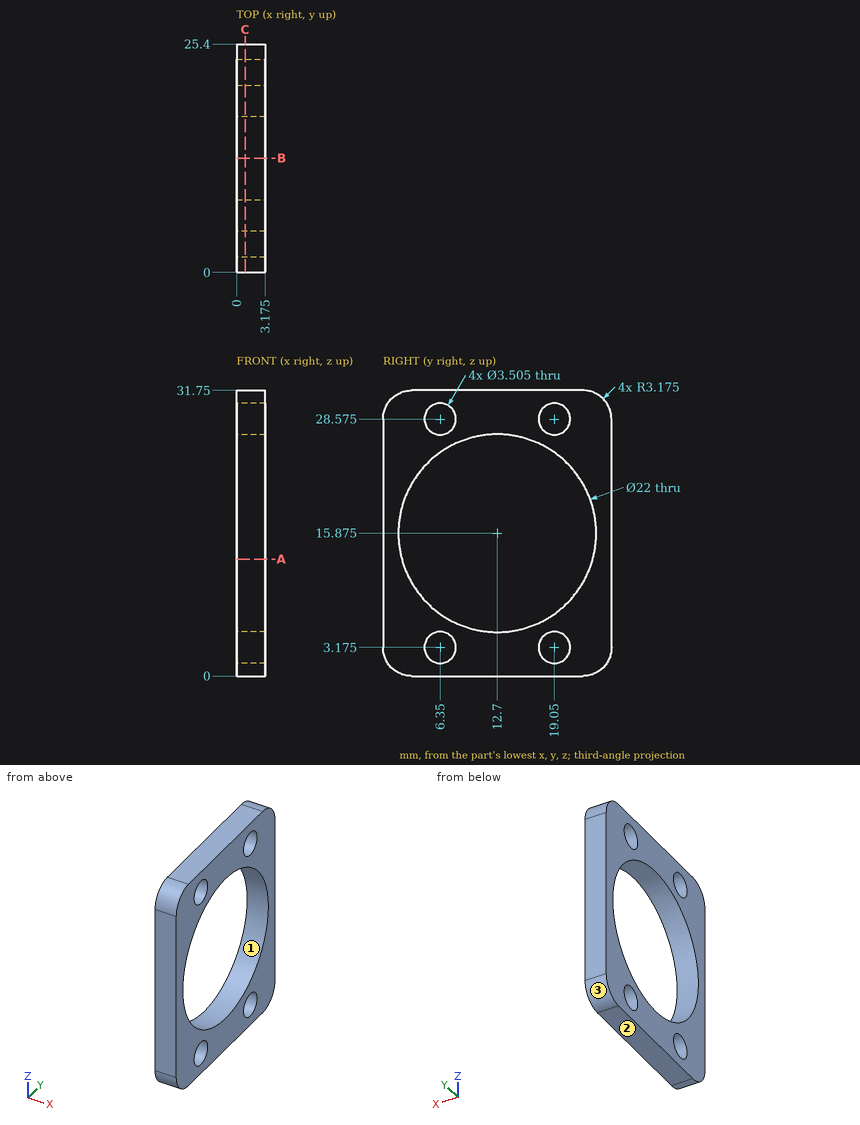
Answer from the drawing. Dimensions are ordinates in mm from the lowest x, y and z of the part. Coordinates: 2 decimals unless noted, no trailing zeros. Write each loop counter-clockwise with the first axis right and the second up, starting at its lowest first coordinate (ties: lowest second). Pieces come first, ordered by that corner, then holes. Notation, with made-up numbers: M 66.5,-36.5 L 109.5,-36.5 A13 ccw 109.5,-28.5 Z; hole C 36,63 d8. An arc over 180 degrees is marked long. Put each result on its own line as item: value. Start each with the question number.
1. A cutting plane is placed at B-B on y = 12.7. Write down the section's boundary in (x, z) (3 decimals).
2. A cutting plane is placed at C-C on x = 0.95. Count the separate pieces of the cut face and the enclosed holes in it, then the cut area to 3 significant figures.
3. A cutting plane is placed at A-A on z = 13. Write down the section's boundary in (x, y) (1 decimal), then the cut area to 3 significant figures.
4. For a pull along Y with two mould halves and no side action, classify the marked faces 1, 2 and 3 as pulls with the +Y half, pulls with the -Y half, needs draft (parallel to the pull), parting line crosses it, or undercut.
5. Consider line 1 (Y direction, x = 2.4, z = 28.5); line 2 (Z direction, x = 2.25, y = 6.35); line 3 (Z direction, x = 2.3, y = 12.5). Determine where each line is inside the solid, lowest interval first. Write a range as from..to.
Resolved:
1. outline: M 0,0 L 3.175,0 L 3.175,4.875 L 0,4.875 Z; M 0,26.875 L 3.175,26.875 L 3.175,31.75 L 0,31.75 Z
2. separate pieces: 1
2. enclosed holes: 5
2. area: 379 mm2
3. outline: M 0,0 L 3.2,0 L 3.2,2.1 L 0,2.1 Z; M 0,23.3 L 3.2,23.3 L 3.2,25.4 L 0,25.4 Z
3. area: 13.2 mm2
4. face 1: undercut
4. face 2: needs draft
4. face 3: pulls with the +Y half
5. line 1: y = 0..4.6, 8.1..17.3, 20.8..25.4
5. line 2: z = 0..1.42, 4.93..6.89, 24.86..26.82, 30.33..31.75
5. line 3: z = 0..4.88, 26.87..31.75
